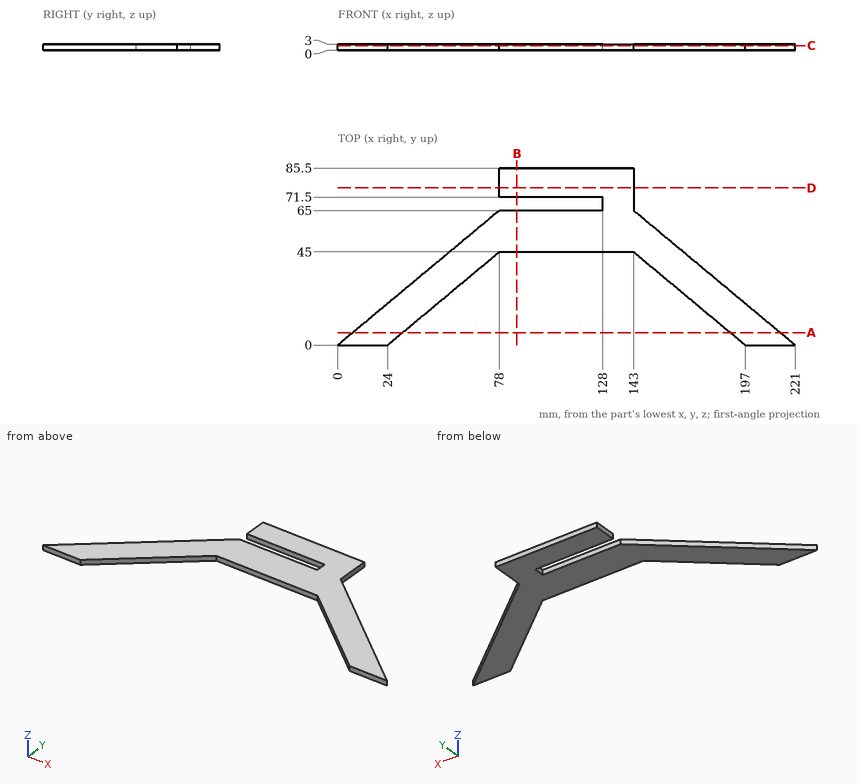
Design review of the part shown in the three views and the two pictorial views. Dimensions are in mm from the part's minimum x, y and z. Give positions to 0.01 mm unless a question says otherwise; leave off trailing zeros. Order: outer loops, then holes, each group sorted by start corner. A loop starts at its lowest first (then second) coordinate and runs counter-clockwise, first axis right, second up. Notation, with made-up numbers: M 1,69.5 L 15,69.5 A20 ccw 15,90.5 Z; hole C -37.75,-12 d6. An arc over 180 degrees is marked long. Answer in a Markdown table with one row per item. Add a question column.
(1) Consider section C-C on z = 2.25. State the section outline as (x, y) points.
(2) Consider section B-B on x = 86.5. State the section outline as (y, z) points.
(3) Consider section A-A on y = 6. State the section outline as (x, z) points.
(4) Wall thickness on probe 1 along Y at (x, z) = (98, 2.05); probe 2 along X at (y, z) = (4.5, 2.5); probe 3 along X at (y, z) = (75.5, 1.7): over which ranges is each line inside the solid? List them lowest first. Write a range as [from, to].
(5) For pin 1 (1.5 mm diameter, centred on x = 102, z = 2, fed in from -Y); pin 2 (1 mm diameter, centred on y = 56, z = 2.5, fed in from +X); pin 3 (0.9 mm diameter, centred on y = 78.5, z = 2, fed in from +X), all flat-tipped, find the tip position at first contact; note any pin that passes through.
(6) Consider section D-D on y = 76. State the section outline as (x, z) points, and give its area (3 significant figures).
Evaluation:
| question | item | result |
|---|---|---|
| 1 | outline | M 0,0 L 24,0 L 78,45 L 143,45 L 197,0 L 221,0 L 143,65 L 143,85.5 L 78,85.5 L 78,71.5 L 128,71.5 L 128,65 L 78,65 Z |
| 2 | outline | M 45,0 L 65,0 L 65,3 L 45,3 Z; M 71.5,0 L 85.5,0 L 85.5,3 L 71.5,3 Z |
| 3 | outline | M 7.2,0 L 31.2,0 L 31.2,3 L 7.2,3 Z; M 189.8,0 L 213.8,0 L 213.8,3 L 189.8,3 Z |
| 4 | probe 1 | y = [45, 65], [71.5, 85.5] |
| 4 | probe 2 | x = [5.4, 29.4], [191.6, 215.6] |
| 4 | probe 3 | x = [78, 143] |
| 5 | pin 1 | stops at y = 45 |
| 5 | pin 2 | stops at x = 154.4 |
| 5 | pin 3 | stops at x = 143 |
| 6 | outline | M 78,0 L 143,0 L 143,3 L 78,3 Z |
| 6 | area | 195 mm^2 |
